The listing builds one solid part. Answer for the finished solid, in the listing's coordinates (mm). Face numbers are marked on the shaded views. A direction names the side the tool comes from. Give positions to 0.01 mm unless a question says otherwise; leave off trailing zeros. Loops run counter-clockwise (first coordinate to the right, second up) from the corner with the lowest first, then second, coordinate; pieces in that order, holes last. Notation, with made-up numbers: (-5, -37) - (18, -37) arc R23 ccw to (18, -2) - close; hole circle Ø8 at (56, 64). An arc over 180 degrees is marked (long way). One line per item, written item: value. Start each with the question number.
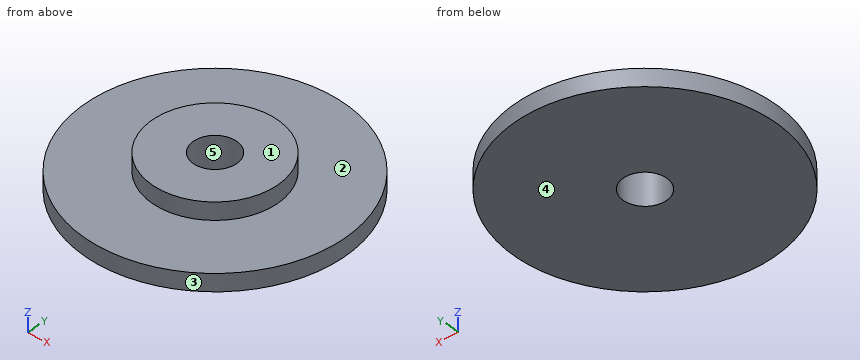
from build123d import *

# Parameters (mm, degrees)
SKETCH1_R           = 47.625
BOSS_EXTRUDE1_DEPTH = 6.35
SKETCH2_R           = 23.0251
BOSS_EXTRUDE2_DEPTH = 6.35
SKETCH4_R           = 7.9375
CUT_EXTRUDE2_DEPTH  = 69.538830235


with BuildPart() as part:
    # Sketch1 → Boss-Extrude1 (new body)
    with BuildSketch(Plane.XY):
        Circle(SKETCH1_R)
    extrude(amount=BOSS_EXTRUDE1_DEPTH)

    # Sketch2 → Boss-Extrude2 (add)
    with BuildSketch(Plane.XY.offset(6.35)):
        Circle(SKETCH2_R)
    extrude(amount=BOSS_EXTRUDE2_DEPTH)

    # Sketch4 → Cut-Extrude2 (cut, through all)
    with BuildSketch(Plane.XY):
        Circle(SKETCH4_R)
    extrude(amount=CUT_EXTRUDE2_DEPTH, mode=Mode.SUBTRACT)


solid = part.part
1. Find the intervals of material crossed by L1, parallel to Y at x = 0, z = 7.25; L2, parallel to Y at x = 0, z = 5 (1 decimal); L3, parallel to Z at x = -8, y = -37, in increasing order. Write a range as [from, to].
2. Determine the mould class of the marked faces 3, 4 and 5 for opening direction Y: released by +Y, released by -Y, zero draft, split by the parting line, or undercut.
3. Flat-ended cylindrical pins translate along their axes: pin 1 (3 mm diameter, centred on y = -11, z = 10.5, fed in from +X); pin 2 (14.5 mm diameter, centred on x = 0, y = 0, fed in from -Z); pin 3 (3 mm diameter, centred on x = -18, z = 4.5, fed in from +Y); pin 4 (2 mm diameter, centred on x = 11.5, z = 7, fed in from -Y). Find the tip coordinate at first contact, or state that the pin passes through.
4. For the marked faces 1 and 2, determine the directions among +Z, -Z, +X, -X, +Y, -Y from which every point of the face is accessible in a straight line to the end or side of a thin tool.
5. A cutting plane is placed at D-D (x = -10). Determine the outline of the cut face in (y, z), plus the area to 3 significant figures.
6. A cutting plane is placed at C-C (z = 7.5). Determine the outline of the cut face in (x, y) (1 decimal), plus the area to 3 significant figures.
Results below:
1. L1: y = [-23.03, -7.94], [7.94, 23.03]
1. L2: y = [-47.6, -7.9], [7.9, 47.6]
1. L3: z = [0, 6.35]
2. face 3: split by the parting line
2. face 4: zero draft
2. face 5: undercut
3. pin 1: stops at x = 20.97
3. pin 2: passes through
3. pin 3: stops at y = 44.68
3. pin 4: stops at y = -46.4
4. face 1: +Z, +X, -X, +Y, -Y
4. face 2: +Z
5. outline: (-46.56, 0) - (46.56, 0) - (46.56, 6.35) - (20.74, 6.35) - (20.74, 12.7) - (-20.74, 12.7) - (-20.74, 6.35) - (-46.56, 6.35) - close
5. area: 855 mm^2
6. outline: circle Ø46.1 at (0, 0); hole circle Ø15.9 at (0, 0)
6. area: 1,470 mm^2
